Verification items for the finished model (mm, model axes). Face numbers are marked on the shaded views. A direction names the side the tool comes from. Round coordinates to 2 decimals unless told otherwise and drop trailing zeros. Order: outer loops, then holes, each group sorted by start corner. A loop starts at its lowest first (then second) coordinate and runs counter-clockwise, first axis right, second up. Notation, with made-up numbers: M 88,-17.75 L 140,-17.75 A12 ccw 140,-3.75 Z; hole C 8,11 d5. An arc over 180 degrees is marked long. Write item = value, one per line. Start each with the question number.
from build123d import *

# Parameters (mm, degrees)
F1_DEPTH = 381
F2_W     = 353.251727
F2_H     = 73.522702
F3_DEPTH = 119.243709
F4_SIZE  = 2.54
F6_D     = 50.8


with BuildPart() as f1:
    # F0 (on Right) → F1 (new body)
    with BuildSketch(Plane.YZ):
        Polygon((22.86, -3.707027), (40.7773, -73.522702), (55.914324, -73.522702), (55.914324, 9.267568), (-63.328385, 9.267568), (-63.328385, -73.522702), (-50.044864, -73.522702), (-31.509727, -3.707027), align=None)
    extrude(amount=F1_DEPTH)

    # F2 (on face) → F3 (cut, through all)
    with BuildSketch(Plane.XZ.offset(63.328385)):
        with Locations((192.336394, -36.761351)):
            Rectangle(F2_W, F2_H)
    extrude(amount=-F3_DEPTH, mode=Mode.SUBTRACT)

    # F4
    f4_edges = [f1.edges().sort_by_distance(p)[0] for p in [
        (381, -3.707031, 9.267568),
        (190.5, -63.328385, 9.267568),
        (190.5, 55.914324, 9.267568),
        (0, -3.707031, 9.267568),
    ]]
    chamfer(f4_edges, length=F4_SIZE)

    # F6 (through all)
    with Locations(Plane.XY.offset(9.267568)):
        with Locations((78.291252, 27.173208), (174.22092, 19.350618), (265.621692, 15.64518)):
            Hole(F6_D / 2)


solid = f1.part
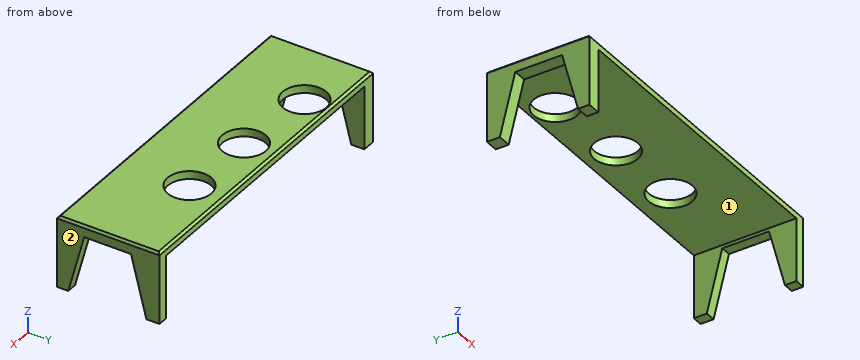
1) Cross-section at D-D, the plane x = 314. Enter the section's corners in (y, z), then the cut area to 3 significant figures.
2) Scan lines: probe 1 along X at (y, z) = (47, -60.5); probe 2 along Z at (x, y) = (155, 47); probe 3 along X at (y, z) = (22, 5). Record each from-to range of solid material in increasing order.
3) Cross-section at A-A, the plane z = -38. Enter the section's corners in (x, y).
4) Access from +Z, -Z, +X, -X, +Y, -Y to the whole of each face (thin tool, end or side, straight path). Record for the marked faces 1 and 2.
5) Cross-section at B-B, the plane x = 266.5. Enter the section's corners in (y, z).
6) Cross-section at C-C, the plane y = -16.5. Enter the section's corners in (x, z).
7) Gauge pin test, flat ends, axial feed: P1, Ø3.5, axis at x = 374, y = -2.5, coming from the -Z side; P2, Ø2, axis at y = 31, z = -40, coming from the -X side. Record the tip position at first contact, or that the pin passes through.
Geometry results:
q1.outline = M -63.33,0 L 55.91,0 L 55.91,6.73 L 53.37,9.27 L -60.79,9.27 L -63.33,6.73 Z
q1.area = 1,100 mm^2
q2.probe_1 = 0 to 15.71, 368.96 to 381
q2.probe_2 = 0 to 9.27
q2.probe_3 = 0 to 53.42, 103.16 to 148.96, 199.48 to 241.03, 290.21 to 381
q3.outline = M 0,-63.33 L 15.71,-63.33 L 15.71,-40.61 L 0,-40.61 Z; M 0,31.66 L 15.71,31.66 L 15.71,55.91 L 0,55.91 Z; M 368.96,-63.33 L 381,-63.33 L 381,-40.61 L 368.96,-40.61 Z; M 368.96,31.66 L 381,31.66 L 381,55.91 L 368.96,55.91 Z
q4.face_1 = -Z, +Y, -Y
q4.face_2 = +Z, -Z, +X, +Y, -Y
q5.outline = M -63.33,0 L -9.74,0 L -9.74,9.27 L -60.79,9.27 L -63.33,6.73 Z; M 41.03,0 L 55.91,0 L 55.91,6.73 L 53.37,9.27 L 41.03,9.27 Z
q6.outline = M 0,-3.71 L 15.71,-3.71 L 15.71,0 L 368.96,0 L 368.96,-3.71 L 381,-3.71 L 381,6.73 L 378.46,9.27 L 2.54,9.27 L 0,6.73 Z
q7.P1 = -3.71
q7.P2 = through
